Geometry check sheet. Reference: the model listing, model coordinates, mm. Face numbers are marked on the shaded views. A direction names the side the tool comes from. Give positions to 0.01 mm unless a question says otherwise; leave off trailing zeros. Loops run counter-clockwise (first coordinate to the right, second up) from the corner with the lowest first, then second, coordinate; pieces in that order, holes last. Notation, with made-up numbers: (-1.5, -3.5) -> (43.5, -3.5) arc R20 cw to (43.5, 3.5) -> close; hole circle Ø6 at (-4, -18.5). An arc over 180 degrees is marked (long way). Write each question's results on one line, items separated by ' | '. Start each with the question number.
1) Sectioned sample at B-B on x = 4. Record the cut outline in (y, z).
2) Scan lines: line 1 (X direction, y = 1.5, z = -14); line 2 (X direction, y = 12.75, z = 21); line 3 (Y direction, x = 30, z = -12). Record each from-to range of solid material in increasing order. Write a range as from..to.
3) Sectioned sample at A-A on z = -13.5. Record the cut outline in (x, y), then the cut area to 3 significant figures.
4) Sectioned sample at D-D on y = 11.25. Record the cut outline in (x, z), then the cut area to 3 significant figures.
5) Set-up check for the marked faces 1 and 2: record each of +Z, -Z, +X, -X, +Y, -Y from which the full face is reachable in a straight line by a thin tool's end or side.
6) Depth check by flat-ended pin: pin 1 (0.5 mm diameter, centred on x = 45.5, z = -9.5, fed in from +Y); pin 2 (0.5 mm diameter, centred on x = 45.5, y = 9, fed in from -Z); pin 3 (0.8 mm diameter, centred on x = 45.5, y = 14.5, fed in from +Z). Enter the tip coordinate at first touch or a pass-through.
7) Sectioned sample at C-C on y = 1.75. Record the cut outline in (x, z).
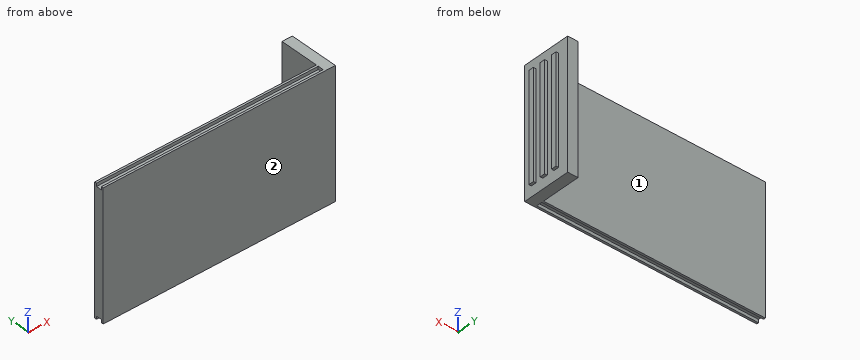
```python
from build123d import *

# Parameters (mm, degrees)
SKETCH1_W           = 90
SKETCH1_H           = 49.6
BOSS_EXTRUDE1_DEPTH = 3.8
SKETCH2_W           = 1.2
SKETCH2_H           = 2.2
CUT_EXTRUDE1_DEPTH  = 91
SKETCH3_W           = 4
SKETCH3_H           = 49.6
BOSS_EXTRUDE2_DEPTH = 19
SKETCH4_W           = 41.6
SKETCH4_H           = 2
BOSS_EXTRUDE3_DEPTH = 1
LPATTERN1_COUNT     = 3
LPATTERN1_PITCH     = 5


with BuildPart() as part:
    # Sketch1 → Boss-Extrude1 (new body)
    with BuildSketch(Plane(origin=(0, 0, 0), x_dir=(1, 0, 0), z_dir=(0, 1, 0))):
        Rectangle(SKETCH1_W, SKETCH1_H)
    extrude(amount=BOSS_EXTRUDE1_DEPTH)

    # Sketch2 → Cut-Extrude1 (cut, through all)
    with BuildSketch(Plane(origin=(45, 0, 0), x_dir=(0, 0, -1), z_dir=(1, 0, 0))):
        with Locations((-24.2, 1.9)):
            Rectangle(SKETCH2_W, SKETCH2_H)
    cut_extrude1 = extrude(amount=-CUT_EXTRUDE1_DEPTH, mode=Mode.SUBTRACT)

    # Mirror1: Cut-Extrude1 across plane
    add(cut_extrude1.mirror(Plane.XY), mode=Mode.SUBTRACT)

    # Sketch3 → Boss-Extrude2 (add)
    with BuildSketch(Plane.XZ):
        with Locations((43, 0)):
            Rectangle(SKETCH3_W, SKETCH3_H)
    extrude(amount=-BOSS_EXTRUDE2_DEPTH)

    # Sketch4 → Boss-Extrude3 (add)
    with BuildSketch(Plane(origin=(45, 0, 0), x_dir=(0, 0, -1), z_dir=(1, 0, 0))):
        with Locations((0, 14)):
            Rectangle(SKETCH4_W, SKETCH4_H)
    boss_extrude3 = extrude(amount=BOSS_EXTRUDE3_DEPTH)

    # LPattern1: Boss-Extrude3 ×3
    with Locations(*[(0, -i * LPATTERN1_PITCH, 0) for i in range(1, LPATTERN1_COUNT)]):
        add(boss_extrude3)


solid = part.part
```
Result:
1) outline: (0, -24.8) -> (0.8, -24.8) -> (0.8, -23.6) -> (3, -23.6) -> (3, -24.8) -> (3.8, -24.8) -> (3.8, 24.8) -> (3, 24.8) -> (3, 23.6) -> (0.8, 23.6) -> (0.8, 24.8) -> (0, 24.8) -> close
2) line 1: -45..45 | line 2: 41..45 | line 3: 0..3.8
3) outline: (-45, 0) -> (45, 0) -> (45, 3) -> (46, 3) -> (46, 5) -> (45, 5) -> (45, 8) -> (46, 8) -> (46, 10) -> (45, 10) -> (45, 13) -> (46, 13) -> (46, 15) -> (45, 15) -> (45, 19) -> (41, 19) -> (41, 3.8) -> (-45, 3.8) -> close | area: 409 mm^2
4) outline: (41, -24.8) -> (45, -24.8) -> (45, 24.8) -> (41, 24.8) -> close | area: 198 mm^2
5) face 1: +Z, -Z, -X, +Y | face 2: +Z, -Z, +X, -X, -Y
6) pin 1: y = 15 | pin 2: z = -20.8 | pin 3: z = 20.8
7) outline: (-45, -23.6) -> (41, -23.6) -> (41, -24.8) -> (45, -24.8) -> (45, 24.8) -> (41, 24.8) -> (41, 23.6) -> (-45, 23.6) -> close
